```python
from build123d import *

# Parameters (mm, degrees)
SKETCH1_R           = 5
SKETCH1_R_2         = 15
BOSS_EXTRUDE1_DEPTH = 90
SKETCH2_W           = 25
SKETCH2_H           = 20
SKETCH2_H_2         = 30
CUT_EXTRUDE1_DEPTH  = 61
FILLET1_R           = 5


with BuildPart() as part:
    # Sketch1 → Boss-Extrude1 (new body)
    with BuildSketch(Plane(origin=(0, 0, 0), x_dir=(1, 0, 0), z_dir=(0, 1, 0))):
        with BuildLine():
            Line((30, 0), (30, 32.5))
            ThreePointArc((30, 32.5), (27.071067812, 39.571067812), (20, 42.5))
            Line((20, 42.5), (-20, 42.5))
            ThreePointArc((-20, 42.5), (-27.071067812, 39.571067812), (-30, 32.5))
            Line((-30, 32.5), (-30, 0))
            Line((-30, 0), (-30, -13.012820513))
            Line((-30, -13.012820513), (-22.471910112, -28.45505618))
            ThreePointArc((-22.471910112, -28.45505618), (0, -42.5), (22.471910112, -28.45505618))
            Line((22.471910112, -28.45505618), (30, -13.012820513))
            Line((30, -13.012820513), (30, 0))
        make_face()
        with Locations((-15, 32.5)):
            Circle(SKETCH1_R, mode=Mode.SUBTRACT)
        with Locations((15, 32.5)):
            Circle(SKETCH1_R, mode=Mode.SUBTRACT)
        with Locations((0, -17.5)):
            Circle(SKETCH1_R_2, mode=Mode.SUBTRACT)
    extrude(amount=BOSS_EXTRUDE1_DEPTH)

    # Sketch2 → Cut-Extrude1 (cut, through all)
    with BuildSketch(Plane(origin=(30, 0, 0), x_dir=(0, 0, -1), z_dir=(1, 0, 0))):
        with BuildLine():
            Line((-42.5, 80), (6.5, 80))
            ThreePointArc((6.5, 80), (7.207106781, 79.707106781), (7.5, 79))
            Line((7.5, 79), (7.5, 11))
            ThreePointArc((7.5, 11), (7.207106781, 10.292893219), (6.5, 10))
            Line((6.5, 10), (-42.5, 10))
            Line((-42.5, 10), (-42.5, 80))
        make_face()
        with Locations((30, 80)):
            Rectangle(SKETCH2_W, SKETCH2_H)
        with Locations((30, 10)):
            Rectangle(SKETCH2_W, SKETCH2_H)
        with Locations((30, 45)):
            Rectangle(SKETCH2_W, SKETCH2_H_2)
    extrude(amount=-CUT_EXTRUDE1_DEPTH, mode=Mode.SUBTRACT)

    # Fillet1
    fillet1_edges = [part.edges().sort_by_distance(p)[0] for p in [
        (0, 0, -17.5),
        (0, 90, -17.5),
    ]]
    fillet(fillet1_edges, radius=FILLET1_R)


solid = part.part
```
The model under review builds one solid part; all positions refer to its coordinate system, in mm. A direction names the side the tool comes from. Give positions to 0.01 mm unless a question says otherwise; leave off trailing zeros. Loops run counter-clockwise (first coordinate to the right, second up) from the corner with the lowest first, then second, coordinate; pieces in that order, holes last. Notation, with made-up numbers: (-24, 26) - (19, 26) arc R29 cw to (19, 61) - close; hole circle Ø3 at (-6.5, -11). An arc over 180 degrees is marked (long way). Answer as a JSON object with one key per item and string values.
Q1. Insertion check: pin 1 (12 mm diameter, centred on x = 8.5, y = 11.5, fed in from -Z); pin 2 (13 mm diameter, centred on x = -15, z = -32.5, fed in from +Y). Each pin has a flat end and moves straight along its axis. Give the tip position at first contact, or say it passes through.
Worked out:
{"pin 1": "stops at z = -17.5", "pin 2": "stops at y = 70"}
Q2. Add section D-D on x = 26.5. State the section outline as (y, z) points, plus the area to 3 significant figures.
Worked out:
{"outline": "(0, -12.5) arc R5 ccw to (5, -17.5) - (20, -17.5) - (20, -40.1) - (30, -40.1) - (30, -17.5) - (60, -17.5) - (60, -40.1) - (70, -40.1) - (70, -17.5) - (85, -17.5) arc R5 ccw to (90, -12.5) - (90, 20.19) - (80, 20.19) - (80, -6.5) arc R1 cw to (79, -7.5) - (11, -7.5) arc R1 cw to (10, -6.5) - (10, 20.19) - (0, 20.19) - close", "area": "1,900 mm^2"}
Q3. Add section B-B on z = -26. State the section outline as (x, y) points.
Worked out:
{"outline": "(-30, 20) - (30, 20) - (30, 30) - (-30, 30) - close; (-30, 60) - (30, 60) - (30, 70) - (-30, 70) - close"}
Q4. Mouldability with a two-part tool opening along Z and no side actions: class faces 1 (the cylindrical face through (19.77, 24.93, -34)), 2 (the cylindrical face through (-26.99, 64.93, -39.65)), 3 (the flat face through (0, 70, -30)) as +Z half, -Z half, draft (parallel to the pull), parting line (faces both ways), or undercut.
Worked out:
{"face 1": "undercut", "face 2": "-Z half", "face 3": "draft"}
Q5. For faces 4 (the flat face through (0, 0, 2)), 5 (the flat face through (0, 12, -17.5)), 6 (the flat face through (0, 60, -30)), 7 (the cylindrical face through (-0.42, 88.57, -16)), 8 (the flat face through (0, 10, 1)), list the 3-axis set-ups (+Z, -Z, +X, -X, +Y, -Y) from which the entire face can be reached by the end or side of a thin tool; tool diameter is ignored.
Worked out:
{"face 4": "+Z, -Z, +X, -X, -Y", "face 5": "-Z, +X, -X, -Y", "face 6": "-Z, +X, -X", "face 7": "-Z, +X, -X, +Y", "face 8": "+Z, +X, -X"}
Q6. To check wall thickness, follow line 1 along Y through (x, z) = (26, -1); line 2 along Y through (x, z) = (-5, -37); line 3 along X through (y, z) = (22, -32). State the ranges of each line that lie inside material, in increasing order.
Worked out:
{"line 1": "y = 0 to 10, 80 to 90", "line 2": "y = 20 to 30, 60 to 70", "line 3": "x = -30 to -19.97, -10.03 to 10.03, 19.97 to 30"}
Q7. Add section C-C on z = 23. State the section outline as (x, y) points, plus the area to 3 significant figures.
Worked out:
{"outline": "(-25.13, 0) - (-13.96, 0) - (-13.96, 10) - (-25.13, 10) - close; (-25.13, 80) - (-13.96, 80) - (-13.96, 90) - (-25.13, 90) - close; (13.96, 0) - (25.13, 0) - (25.13, 10) - (13.96, 10) - close; (13.96, 80) - (25.13, 80) - (25.13, 90) - (13.96, 90) - close", "area": "447 mm^2"}
Q8. Add section A-A on x = 0. State the section outline as (y, z) points.
Worked out:
{"outline": "(0, -12.5) arc R5 ccw to (5, -17.5) - (20, -17.5) - (20, -42.5) - (30, -42.5) - (30, -17.5) - (60, -17.5) - (60, -42.5) - (70, -42.5) - (70, -17.5) - (85, -17.5) arc R5 ccw to (90, -12.5) - (90, 2.5) - (80, 2.5) - (80, -6.5) arc R1 cw to (79, -7.5) - (11, -7.5) arc R1 cw to (10, -6.5) - (10, 2.5) - (0, 2.5) - close; (0, 32.5) - (10, 32.5) - (10, 42.5) - (0, 42.5) - close; (80, 32.5) - (90, 32.5) - (90, 42.5) - (80, 42.5) - close"}
